For this review, use the dimensioned drawing (mm, ordinates from the lowest corner) and the shaded views. Coordinates: 2 decimals unless noted, no trailing zeros. Write each loop counter-clockwise with the first axis right and the second up, starting at its lowest first coordinate (ties: lowest second). Pieces come first, ordered by that corner, then holes. Notation, with made-up numbers: (72.5, 14) -> (130.5, 14) arc R22 cw to (130.5, 46) -> close; hole circle Ø10 at (16.5, 4.5). An arc over 180 degrees is marked (long way). Put each result on its own line as item: value. Start each with the question number.
Item 1: Consider section D-D on x = 15.5. Give the boundary of the cut face in (y, z).
Item 2: Insertion check: P1, Ø2, axis at x = 11, y = 20, coming from the +Z side; P2, Ø2.5, axis at x = 11, y = 11, coming from the +Z side; P3, Ø1, axis at y = 13, z = 1, coming from the +X side; P4, Ø0.6, axis at y = 11.5, z = 1, coming from the -X side. Each pin has a flat end and moves straight along its axis. Give the tip position at first contact, or say it passes through.
Item 3: To check wall thickness, follow L1, parallel to Y at x = 11, z = 1.4; L2, parallel to X at y = 6.5, z = 1.4; L3, parallel to X at y = 10.75, z = 0.65. State the ranges of each line that lie inside material, in increasing order.
Item 4: Consider section A-A on y = 11. Give the boundary of the cut face in (x, z), and give its area (3 significant figures).
Item 5: Consider section B-B on z = 1.5. Give the boundary of the cut face in (x, y).
Item 6: Consider section C-C on x = 11. Give the boundary of the cut face in (y, z).
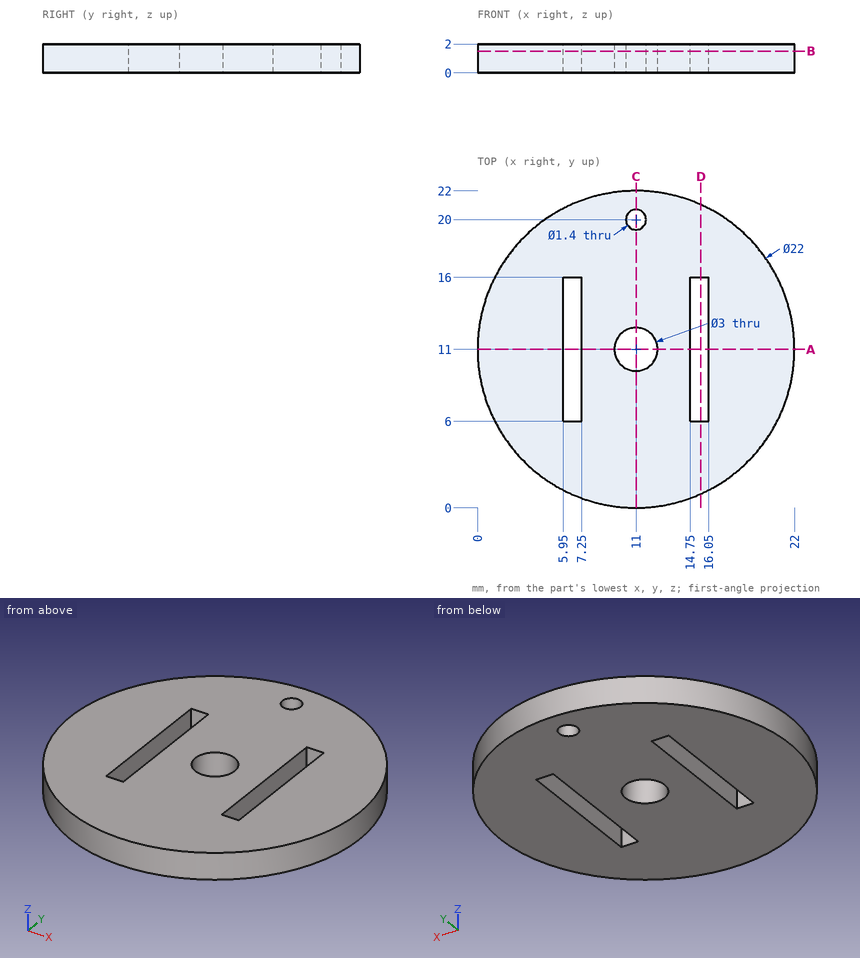
Return value:
1. outline: (0.96, 0) -> (6, 0) -> (6, 2) -> (0.96, 2) -> close; (16, 0) -> (21.04, 0) -> (21.04, 2) -> (16, 2) -> close
2. P1: z = 2
2. P2: through
2. P3: x = 21.9
2. P4: x = 0
3. L1: 0 to 9.5, 12.5 to 19.3, 20.7 to 22
3. L2: 0.96 to 5.95, 7.25 to 14.75, 16.05 to 21.04
3. L3: 0 to 5.95, 7.25 to 9.52, 12.48 to 14.75, 16.05 to 22
4. outline: (0, 0) -> (5.95, 0) -> (5.95, 2) -> (0, 2) -> close; (7.25, 0) -> (9.5, 0) -> (9.5, 2) -> (7.25, 2) -> close; (12.5, 0) -> (14.75, 0) -> (14.75, 2) -> (12.5, 2) -> close; (16.05, 0) -> (22, 0) -> (22, 2) -> (16.05, 2) -> close
4. area: 32.8 mm^2
5. outline: circle Ø22 at (11, 11); hole (5.95, 6) -> (7.25, 6) -> (7.25, 16) -> (5.95, 16) -> close; hole circle Ø3 at (11, 11); hole circle Ø1.4 at (11, 20); hole (14.75, 6) -> (16.05, 6) -> (16.05, 16) -> (14.75, 16) -> close
6. outline: (0, 0) -> (9.5, 0) -> (9.5, 2) -> (0, 2) -> close; (12.5, 0) -> (19.3, 0) -> (19.3, 2) -> (12.5, 2) -> close; (20.7, 0) -> (22, 0) -> (22, 2) -> (20.7, 2) -> close
